Geometry check sheet. Reference: the model listing, model coordinates, mm. Face numbers are marked on the shaded views. A direction names the side the tool comes from. Round coordinates to 2 decimals unless told otherwise and drop trailing zeros. Write each loop counter-clockwise with the first axis right and the second up, starting at its lowest first coordinate (ties: lowest second). Pieces come first, ordered by that corner, then holes.
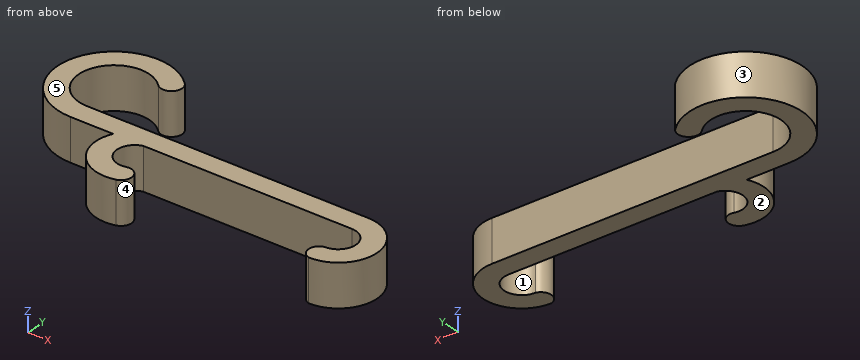
from build123d import *

# Parameters (mm, degrees)
F1_DEPTH = 6


with BuildPart() as f1:
    # F0 (on Top) → F1 (new body)
    with BuildSketch(Plane.XY):
        with BuildLine():
            ThreePointArc((40, -10.917138), (45.458569, -5.458569), (40, 0))
            Line((40, 0), (10.035747, 0))
            ThreePointArc((10.035747, 0), (7.687968, -1.023864), (6.058475, -3))
            Line((6.058475, -3), (10.352952, -3))
            Line((10.352952, -3), (40, -3))
            ThreePointArc((40, -3), (42.5, -5.5), (40, -8))
            ThreePointArc((40, -8), (38.85671, -9.458569), (40, -10.917138))
        make_face()
        with BuildLine():
            ThreePointArc((6.058475, -3), (7.687968, -1.023864), (10.035747, 0))
            Line((10.035747, 0), (0, 0))
            ThreePointArc((0, 0), (-4.619398, 6.913417), (3.535534, 8.535534))
            ThreePointArc((3.535534, 8.535534), (5.656854, 8.535534), (5.656854, 10.656854))
            ThreePointArc((5.656854, 10.656854), (-7.391036, 8.061467), (0, -3))
            Line((0, -3), (6.058475, -3))
        make_face()
        with BuildLine():
            Line((10.352952, -3), (6.058475, -3))
            ThreePointArc((6.058475, -3), (6.75473, -8.911625), (12.423505, -10.727407))
            ThreePointArc((12.423505, -10.727407), (13.484165, -8.890289), (11.647048, -7.829629))
            ThreePointArc((11.647048, -7.829629), (8.585185, -6.061862), (10.352952, -3))
        make_face()
    extrude(amount=F1_DEPTH)


solid = f1.part
1. Depth check by flat-ended pin: pin 1 Ø12 at (x, y) = (36.5, 8) entering from -Z; pin 2 Ø13 at (x, y) = (0, 5) entering from +Z; pin 3 Ø1 at (x, z) = (-1, 1.5) entering from -Y; pin 4 Ø3 at (x, z) = (5.5, 3) entering from -Y. Enter the tip coordinate at first touch or a pass-through.
2. Access from +Z, -Z, +X, -X, +Y, -Y to the whole of each face (thin tool, end or side, straight path). Record for the marked faces 1 and 2.
3. Release check for a two-part mould opening along X. For the marked faces 3, 4 and 5 record: +X half, -X half, draft (parallel to the pull), parting line (faces both ways), or undercut.
4. Section check A-A (x = 11). Record the cut outline in (y, z), plus the area to 3 significant figures.
5. Section check B-B (y = 9.25). Record the cut outline in (x, z), plus the area to 3 significant figures.
6. Section check C-C (x = 22.5). Record the cut outline in (y, z).
7. Section check D-D (z = 1.8). Record the cut outline in (x, y), plus the area to 3 significant figures.
8. Scan lines: line 1 along Y through (x, z) = (0, 3.8); line 2 along X through (y, z) = (-5.5, 1.9); line 3 along X through (y, z) = (5, 4.5). Record each from-to range of solid material in increasing order.
Results below:
1. pin 1: passes through
1. pin 2: stops at z = 6
1. pin 3: stops at y = -2.98
1. pin 4: stops at y = -9.19
2. face 1: +Z, -Z
2. face 2: -Z, +X, -X, +Y, -Y
3. face 3: parting line
3. face 4: undercut
3. face 5: draft
4. outline: (-10.91, 0) - (-7.91, 0) - (-7.91, 6) - (-10.91, 6) - close; (-3, 0) - (0, 0) - (0, 6) - (-3, 6) - close
4. area: 36.0 mm2
5. outline: (-6.78, 0) - (-2.63, 0) - (-2.63, 6) - (-6.78, 6) - close; (2.63, 0) - (6.06, 0) - (6.06, 6) - (2.63, 6) - close
5. area: 45.4 mm2
6. outline: (-3, 0) - (0, 0) - (0, 6) - (-3, 6) - close
7. outline: (0, -3) - (6.06, -3) arc R5.5 ccw to (12.42, -10.73) arc R1.5 ccw to (11.65, -7.83) arc R2.5 cw to (10.35, -3) - (40, -3) arc R2.5 cw to (40, -8) arc R1.5 ccw to (40, -10.92) arc R5.46 ccw to (40, 0) - (0, 0) arc R5 cw (long way) to (3.54, 8.54) arc R1.5 ccw to (5.66, 10.66) arc R8 ccw (long way) to start
7. area: 273 mm2
8. line 1: y = -3 to 0, 10 to 13
8. line 2: x = 5.5 to 8.5, 42.5 to 45.46
8. line 3: x = -8 to -5
